```python
from build123d import *

# Parameters (mm, degrees)
BOSS_EXTRUDE1_DEPTH = 10
SKETCH2_R           = 2
BOSS_EXTRUDE2_DEPTH = 30


with BuildPart() as part:
    # Sketch1 → Boss-Extrude1 (new body)
    with BuildSketch(Plane(origin=(0, 0, 0), x_dir=(1, 0, 0), z_dir=(0, 1, 0))):
        with BuildLine():
            Line((-4.915670141, -9.915670141), (12.084329859, -9.915670141))
            ThreePointArc((12.084329859, -9.915670141), (13.498543421, -9.329883704), (14.084329859, -7.915670141))
            Line((14.084329859, -7.915670141), (14.084329859, -0.738316599))
            ThreePointArc((14.084329859, -0.738316599), (12.841308154, 2.560943028), (9.730284223, 4.219782125))
            Line((9.730284223, 4.219782125), (2.224360471, 4.219782125))
            ThreePointArc((2.224360471, 4.219782125), (0.833058018, 4.022310364), (-0.448347257, 3.445493118))
            Line((-0.448347257, 3.445493118), (-8.984753233, -1.953673617))
            ThreePointArc((-8.984753233, -1.953673617), (-9.667550015, -2.67911766), (-9.915670141, -3.643958014))
            Line((-9.915670141, -3.643958014), (-9.915670141, -4.915670141))
            ThreePointArc((-9.915670141, -4.915670141), (-8.451204047, -8.451204047), (-4.915670141, -9.915670141))
        make_face()
        with BuildLine():
            Line((-6.036927005, -3.259535169), (-1.898433993, -0.45764174))
            ThreePointArc((-1.898433993, -0.45764174), (0.775850036, 0.822194595), (3.707850327, 1.261683401))
            Line((3.707850327, 1.261683401), (9.084329859, 1.261683401))
            ThreePointArc((9.084329859, 1.261683401), (11.084329859, -0.738316599), (9.084329859, -2.738316599))
            Line((9.084329859, -2.738316599), (4.908888201, -2.738316599))
            ThreePointArc((4.908888201, -2.738316599), (1.976887911, -3.177805405), (-0.697396118, -4.45764174))
            Line((-0.697396118, -4.45764174), (-3.604145519, -6.425604963))
            ThreePointArc((-3.604145519, -6.425604963), (-6.501561039, -6.134255412), (-6.036927005, -3.259535169))
        make_face(mode=Mode.SUBTRACT)
    extrude(amount=BOSS_EXTRUDE1_DEPTH)

    # Sketch2 → Boss-Extrude2 (add)
    with BuildSketch(Plane(origin=(14.084329859, 0, 0), x_dir=(0, 0, -1), z_dir=(1, 0, 0))):
        with Locations(Location((-4.833857575, 5, 0), (0, 0, 180))):
            Circle(SKETCH2_R)
    extrude(amount=BOSS_EXTRUDE2_DEPTH)


solid = part.part
```
Model file for the job. Use its own axes, mm. A direction names the side the tool comes from. Give positions to 0.01 mm unless a question says otherwise; leave off trailing zeros. Write each loop counter-clockwise with the first axis right and the second up, starting at its lowest first coordinate (ties: lowest second). Pieces come first, ordered by that corner, then holes. Notation, with made-up numbers: M -20.75,73 L 30.25,73 A34 ccw 30.25,110 Z; hole C 85.5,28 d9. An arc over 180 degrees is marked long. Use a Markdown table: item, result.
1) Cut at B-B (y = 5). List the corners of the cut face in (x, z).
Responses:
| item | result |
|---|---|
| outline | M -9.92,3.64 A2 ccw -8.98,1.95 L -0.45,-3.45 A5 ccw 2.22,-4.22 L 9.73,-4.22 A5 ccw 14.08,0.74 L 14.08,2.83 L 44.08,2.83 L 44.08,6.83 L 14.08,6.83 L 14.08,7.92 A2 ccw 12.08,9.92 L -4.92,9.92 A5 ccw -9.92,4.92 Z; hole M -6.04,3.26 L -1.9,0.46 A10 ccw 3.71,-1.26 L 9.08,-1.26 A2 ccw 9.08,2.74 L 4.91,2.74 A10 cw -0.7,4.46 L -3.6,6.43 A2 ccw long Z |
2) Pull direction Z, two halves, no side cores. Call faces 4 (the flat face through (6, 5, -4.22)), 5 (the cylindrical face through (-8.5, 4.9, 8.4)), 6 (the cylindrical face through (-6.473, 4.93, 6.17)): +Z half, -Z half, draft (parallel to the pull), parting line (faces both ways), or undercut.
Responses:
| item | result |
|---|---|
| face 4 | -Z half |
| face 5 | +Z half |
| face 6 | undercut |
3) Tool access for faces 1 (the cylindrical face through (2.017, 4.93, 3.166)), 2 (the cylindrical face through (28.87, 6.22, 3.25)), 3 (the cylindrical face through (0.852, 4.93, -4.028)): list every direction of +Z, -Z, +X, -X, +Y, -Y with a clear straight run to the whole face (end or side of a thin tool).
Responses:
| item | result |
|---|---|
| face 1 | +Y, -Y |
| face 2 | +X |
| face 3 | -Z, -X, +Y, -Y |
4) Drill centre lines: line 1 (Z direction, x = -1, y = 6.5); line 2 (Z direction, x = -1.5, y = 9); line 3 (X direction, y = 9, z = 6.25). Where is each one in solid material? Low to high. Write a range as from..to.
Responses:
| item | result |
|---|---|
| line 1 | z = -3.1..-0.08, 4.66..9.92 |
| line 2 | z = -2.78..0.2, 5..9.92 |
| line 3 | x = -9.73..-6.41, -3.34..14.08 |
5) Pin check, flat tips, straight feed: pin 1 (5 mm diameter, centred on x = 32, y = 2.5, fed in from -Z); pin 2 (1 mm diameter, centred on x = 29, z = 2, fed in from -Y); pin 3 (6 mm diameter, centred on x = 27, z = 6.5, fed in from -Y); pin 4 (6 mm diameter, centred on x = 20.5, z = 6, fed in from +Y). Stop position of each tip, or through.
Responses:
| item | result |
|---|---|
| pin 1 | stops at z = 2.83 |
| pin 2 | passes through |
| pin 3 | stops at y = 3 |
| pin 4 | stops at y = 7 |
6) Cut at C-C (z = 0). List the corners of the cut face in (x, y).
Responses:
| item | result |
|---|---|
| outline | M -5.9,0 L -1.15,0 L -1.15,10 L -5.9,10 Z; M 10.94,0 L 14.03,0 L 14.03,10 L 10.94,10 Z |
7) Cut at D-D (x = 26.5). List the corners of the cut face in (y, z), and give its area (3 significant figures).
Responses:
| item | result |
|---|---|
| outline | C 5,4.83 d4 |
| area | 12.6 mm2 |
8) Cut at A-A (x = 6). List the corners of the cut face in (y, z), and give its area (3 significant figures).
Responses:
| item | result |
|---|---|
| outline | M 0,-4.22 L 10,-4.22 L 10,-1.26 L 0,-1.26 Z; M 0,2.74 L 10,2.74 L 10,9.92 L 0,9.92 Z |
| area | 101 mm2 |
